Part print with two shaded views. Sizes in mm from the minimum x, y, z corner. A direction names the side the tool comes from. Give positions to 0.01 mm unless a question says otherwise; leave off trailing zeros. Loops run counter-clockwise (first coordinate to the right, second up) from the corner with the lowest first, then second, coordinate; pieces in that order, holes last. Notation, with made-up numbers: (-34.75, 67) -> (0.25, 67) arc R26 cw to (0.25, 86) -> close; hole circle Ø9 at (60, -31.75). An arc over 180 degrees is marked (long way). One line per question, with ' | ' between items.
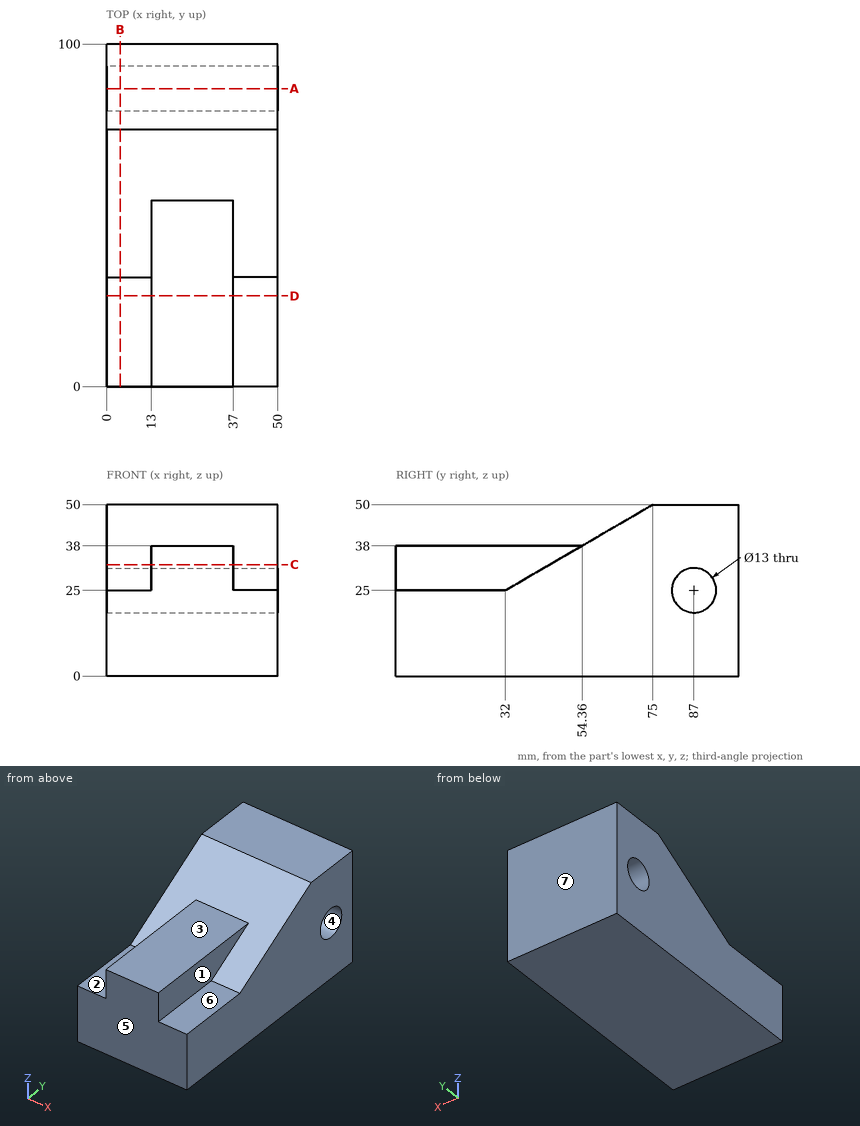
1) Pull direction Y, two halves, no side cores. Call the marked faces 4, 5, 6 and 7: pulls with the +Y half, pulls with the -Y half, needs draft (parallel to the pull), parting line crosses it, or undercut.
Found:
face 4: undercut | face 5: pulls with the -Y half | face 6: needs draft | face 7: pulls with the +Y half
2) Drill centre lines: line 1 (Z direction, x = 11, y = 87); line 2 (Y direction, x = 41, z = 26); line 3 (Z direction, x = 43, y = 11.5). Where is each one in solid material? Low to high.
Found:
line 1: 0 to 18.5, 31.5 to 50 | line 2: 33.72 to 80.58, 93.42 to 100 | line 3: 0 to 25
3) Saw through at D-D (y = 26.5). Give the cut face in (x, z).
Found:
outline: (0, 0) -> (50, 0) -> (50, 25) -> (37, 25) -> (37, 38) -> (13, 38) -> (13, 25) -> (0, 25) -> close
4) Saw through at B-B (x = 4). Give the cut face in (y, z).
Found:
outline: (0, 0) -> (100, 0) -> (100, 50) -> (75, 50) -> (32, 25) -> (0, 25) -> close; hole circle Ø13 at (87, 25)
5) Tool access for the marked faces 1, 2 and 3: list every direction of +Z, -Z, +X, -X, +Y, -Y with a clear straight run to the whole face (end or side of a thin tool).
Found:
face 1: +Z, +X, -Y | face 2: +Z, -X, -Y | face 3: +Z, +X, -X, -Y
6) Pin check, flat tips, straight feed: P1, Ø1.5, axis at x = 26, y = 49.5, coming from the +Z side; P2, Ø4, axis at x = 42.5, y = 20.5, coming from the +Z side; P3, Ø8, axis at y = 87, z = 25, coming from the -X side; P4, Ø5, axis at x = 44, y = 54, coming from the +Z side. Stop position of each tip, or through.
Found:
P1: z = 38 | P2: z = 25 | P3: through | P4: z = 39.24
7) Saw through at A-A (y = 87). Give the cut face in (x, z).
Found:
outline: (0, 0) -> (50, 0) -> (50, 18.5) -> (0, 18.5) -> close; (0, 31.5) -> (50, 31.5) -> (50, 50) -> (0, 50) -> close
8) Saw through at C-C (z = 32.5). Give the cut face in (x, y), and give its area (3 significant figures).
Found:
outline: (0, 44.9) -> (13, 44.9) -> (13, 0) -> (37, 0) -> (37, 44.9) -> (50, 44.9) -> (50, 100) -> (0, 100) -> close | area: 3,830 mm2
